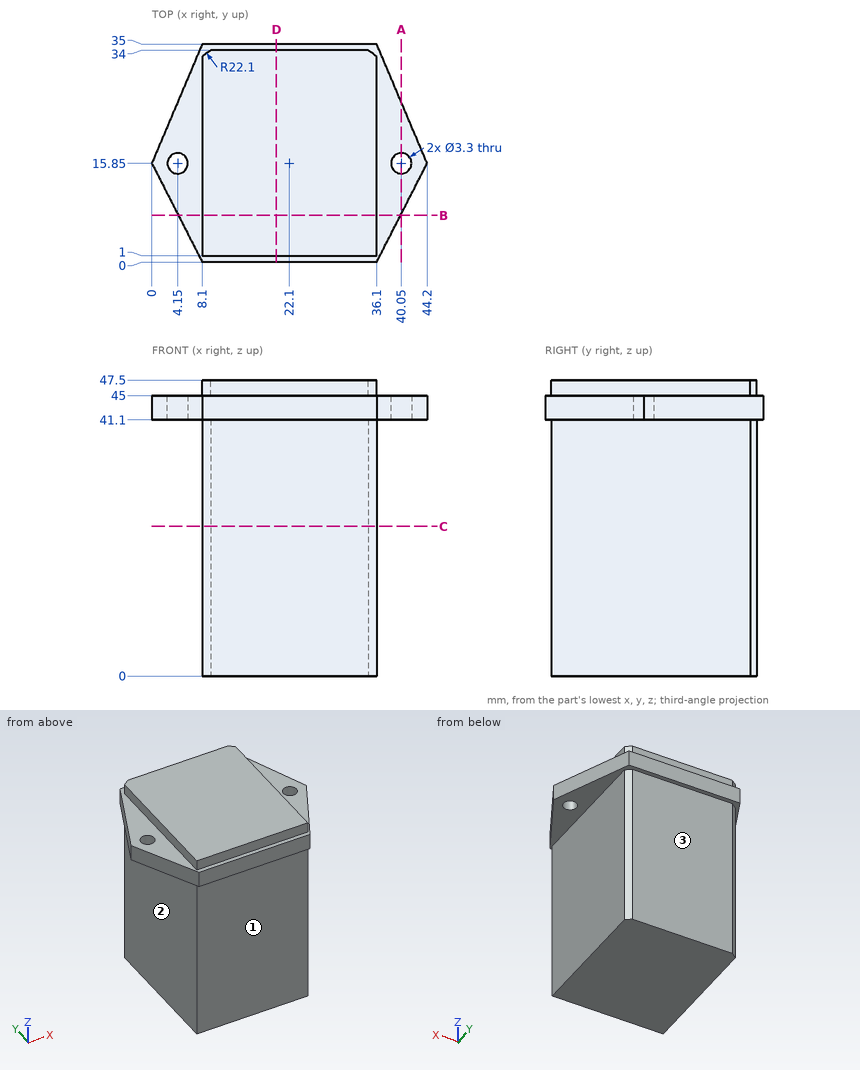
Geometry: see drawing. Coordinates: mm, zero at the bounding-box minimum. A direction names the side the tool comes from. Coordinates: 2 decimals unless noted, no trailing zeros. Loops run counter-clockwise (first coordinate to the right, second up) from the corner with the lowest first, then second, coordinate; pieces in that order, holes last. Notation, with made-up numbers: (7, 42.5) - (40, 42.5) arc R22 cw to (40, 81.5) - close; hole circle Ø5 at (78.5, -2). An arc over 180 degrees is marked (long way). Put each result on its own line as item: value. Start each with the question number.
Q1. Cut plane D-D, the plane x = 20. Return loops of the section in (y, z), and give its area (3 significant figures).
Q2. Line query: line 1 (Y direction, x = 23, z = 24); line 2 (X direction, y = 30.5, z = 8); line 3 (X direction, y = 15, z = 42). Output: solid intervals per line, ascending.
Q3. Cut plane B-B, the plane y = 7.5. Return loops of the section in (x, z).
Q4. Pin query (flat end, axial travel): pin 1 Ø2 at (y, z) = (20.5, 47) entering from +X; pin 2 Ø4 at (x, z) = (35, 23) entering from -Y; pin 3 Ø4.5 at (x, y) = (4.15, 15.85) entering from -Z. Return the tip coordinate at first contact, or that it passes through.
Q5. Set-up query: the marked faces 1, 2 and 3. Return all of +Z, -Z, +X, -X, +Y, -Y with unobstructed straight access to the full face (end or side cutting, diameter ignored); none if empty.
Q6. Cut plane C-C, the plane z = 24. Return loops of the section in (x, y), and give its area (3 significant figures).
Q7. Cut plane A-A, the plane x = 40.05. Return loops of the section in (y, z).
Filled sheet:
1. outline: (0, 41.1) - (1, 41.1) - (1, 0) - (34, 0) - (34, 41.1) - (35, 41.1) - (35, 45) - (34, 45) - (34, 47.5) - (1, 47.5) - (1, 45) - (0, 45) - close
1. area: 1,580 mm²
2. line 1: 1 to 34
2. line 2: 8.1 to 36.1
2. line 3: 0.43 to 2.74, 5.56 to 38.64, 41.46 to 43.77
3. outline: (4.27, 41.1) - (8.1, 41.1) - (8.1, 0) - (36.1, 0) - (36.1, 41.1) - (39.93, 41.1) - (39.93, 45) - (36.1, 45) - (36.1, 47.5) - (8.1, 47.5) - (8.1, 45) - (4.27, 45) - close
4. pin 1: x = 36.1
4. pin 2: y = 1
4. pin 3: z = 41.1
5. face 1: -Z, +X, -X, -Y
5. face 2: -Z, -X, +Y, -Y
5. face 3: -Z, +X, -X, +Y
6. outline: (8.1, 1) - (36.1, 1) - (36.1, 32.95) arc R22.1 ccw to (34.71, 34) - (9.49, 34) arc R22.1 ccw to (8.1, 32.95) - close
6. area: 923 mm²
7. outline: (7.73, 41.1) - (14.2, 41.1) - (14.2, 45) - (7.73, 45) - close; (17.5, 41.1) - (25.66, 41.1) - (25.66, 45) - (17.5, 45) - close
